Autodesk Inventor part; units mm, degrees
ref_plane "YZ Plane" through (0, 0, 0) normal (1, 0, 0) x (0, 1, 0)
ref_plane "XZ Plane" through (0, 0, 0) normal (0, 1, 0) x (-1, 0, 0)
ref_plane "XY Plane" through (0, 0, 0) normal (0, 0, 1) x (1, 0, 0)
sketch "Sketch1" plane through (0, 0, 0) normal (0, 0, 1) x (1, 0, 0)
  line L0 (35.093, -7.2202) -> (-19.907, -7.2202)
  line L1 (-19.907, -7.2202) -> (-19.907, 74.7798)
  line L2 (-19.907, 74.7798) -> (35.093, 74.7798)
  line L3 (35.093, 74.7798) -> (35.093, -7.2202)
  line L4 (-1.6316, 73.7798) -> (15.8684, 73.7798)
  line L5 (15.8684, 73.7798) -> (15.8684, 38.2798)
  line L6 (15.8684, 38.2798) -> (-1.6316, 38.2798)
  line L7 (-1.6316, 38.2798) -> (-1.6316, 73.7798)
  circle A0 centre (7.5885, 28.2798) radius 5.75
  line L8 (12.233, 6.0025) -> (3.233, 6.0025)
  line L9 (3.233, 6.0025) -> (3.233, -3.9975)
  line L10 (3.233, -3.9975) -> (12.233, -3.9975)
  line L11 (12.233, -3.9975) -> (12.233, 6.0025)
  circle A1 centre (7.5885, 28.2798) radius 1.25
  line L12 (3.233, 6.0025) -> (-2.767, 6.0025)
  line L13 (-2.767, 6.0025) -> (-2.767, -3.9975)
  line L14 (-2.767, -3.9975) -> (3.233, -3.9975)
  line L15 (3.233, -3.9975) -> (3.233, 6.0025)
  line L16 (12.233, 5.3167) -> (16.7288, 5.3167)
  line L17 (16.7288, 5.3167) -> (16.7288, 2.7767)
  line L18 (16.7288, 2.7767) -> (12.233, 2.7767)
  line L19 (12.233, 2.7767) -> (12.233, 5.3167)
  line L20 (12.233, -1.5375) -> (12.233, 1.0025)
  line L21 (12.233, -3.4895) -> (12.233, -0.9495)
  line L22 (12.233, 2.2687) -> (16.7288, 2.2687)
  line L23 (16.7288, 2.2687) -> (16.7288, -0.2713)
  line L24 (16.7288, -0.2713) -> (12.233, -0.2713)
  line L25 (12.233, -0.2713) -> (12.233, 2.2687)
  line L26 (12.233, -0.7793) -> (16.7288, -0.7793)
  line L27 (16.7288, -0.7793) -> (16.7288, -3.3193)
  line L28 (16.7288, -3.3193) -> (12.233, -3.3193)
  line L29 (12.233, -3.3193) -> (12.233, -0.7793)
  circle A2 centre (0.233, 0.9987) radius 1.5
  circle A3 centre (0.3684, 66.2798) radius 0.75
  circle A4 centre (0.3684, 63.7398) radius 0.75
  circle A5 centre (0.3684, 61.1998) radius 0.75
  circle A6 centre (0.3684, 58.6598) radius 0.75
  circle A7 centre (0.3684, 56.1198) radius 0.75
  circle A8 centre (0.3684, 53.5798) radius 0.75
  circle A9 centre (0.3684, 51.0398) radius 0.75
  circle A10 centre (0.3684, 48.4998) radius 0.75
  circle A11 centre (13.8684, 63.7398) radius 0.75
  circle A12 centre (13.8684, 58.6598) radius 0.75
  circle A13 centre (13.8684, 56.1198) radius 0.75
  circle A14 centre (13.8684, 53.5798) radius 0.75
  circle A15 centre (13.8684, 48.4998) radius 0.75
  circle A16 centre (13.8684, 66.2798) radius 0.75
  circle A17 centre (13.8684, 51.0398) radius 0.75
  circle A18 centre (13.8684, 61.1998) radius 0.75
  line L30 (-17.907, 69.7798) -> (-16.407, 69.7798)
  line L31 (-16.407, 69.7798) -> (-16.407, -2.2202)
  line L32 (-16.407, -2.2202) -> (-17.907, -2.2202)
  line L33 (-17.907, -2.2202) -> (-17.907, 69.7798)
  line L34 (-15.367, -2.2202) -> (-13.867, -2.2202)
  line L35 (-13.867, -2.2202) -> (-13.867, 69.7798)
  line L36 (-13.867, 69.7798) -> (-15.367, 69.7798)
  line L37 (-15.367, 69.7798) -> (-15.367, -2.2202)
  line L38 (31.593, 69.7798) -> (33.093, 69.7798)
  line L39 (33.093, 69.7798) -> (33.093, -2.2202)
  line L40 (33.093, -2.2202) -> (31.593, -2.2202)
  line L41 (31.593, -2.2202) -> (31.593, 69.7798)
  line L42 (30.553, -2.2202) -> (29.053, -2.2202)
  line L43 (29.053, -2.2202) -> (29.053, 69.7798)
  line L44 (29.053, 69.7798) -> (30.553, 69.7798)
  line L45 (30.553, 69.7798) -> (30.553, -2.2202)
  line L46 (5.8684, 68.7798) -> (10.8684, 68.7798)
  line L47 (10.8684, 68.7798) -> (10.8684, 63.7798)
  line L48 (10.8684, 63.7798) -> (5.8684, 63.7798)
  line L49 (5.8684, 63.7798) -> (5.8684, 68.7798)
  line L50 (6.8684, 55.8198) -> (10.8684, 55.8198)
  line L51 (10.8684, 55.8198) -> (10.8684, 53.2798)
  line L52 (10.8684, 53.2798) -> (6.8684, 53.2798)
  line L53 (6.8684, 53.2798) -> (6.8684, 55.8198)
  line L54 (5.8684, 48.2798) -> (10.8684, 48.2798)
  line L55 (10.8684, 48.2798) -> (10.8684, 43.2798)
  line L56 (10.8684, 43.2798) -> (5.8684, 43.2798)
  line L57 (5.8684, 43.2798) -> (5.8684, 48.2798)
  circle A19 centre (0.8684, 71.2798) radius 1.5
  circle A20 centre (0.8684, 40.7798) radius 1.5
  point P0 (0, 0)
  point P1 (0, 0)
  dimension "d0" = 82
  dimension "d1" = 55
  dimension "d2" = 17.5
  dimension "d3" = 35.5
  dimension "d4" = 11.5
  dimension "d5" = 2.5
  dimension "d6" = 1
  dimension "d7" = 10
  dimension "d8" = 27.4955
  dimension "d9" = 9
  dimension "d10" = 10
  dimension "d11" = 6
  dimension "d12" = 22.86
  dimension "d13" = 19.2246
  dimension "d14" = 2.54
  dimension "d15" = 0.6858
  dimension "d16" = 10
  dimension "d17" = 2.54
  dimension "d18" = 0.508
  dimension "d19" = 4.4958
  dimension "d20" = 4.4958
  dimension "d21" = 2.54
  dimension "d22" = 4.4958
  dimension "d23" = 0.508
  dimension "d24" = 3
  dimension "d25" = 1.5
  dimension "d26" = 7.5
  dimension "d27" = 2
  dimension "d28" = 1.5
  dimension "d29" = 1.5
  dimension "d30" = 1.5
  dimension "d31" = 1.5
  dimension "d32" = 1.5
  dimension "d33" = 1.5
  dimension "d34" = 1.5
  dimension "d35" = 2.54
  dimension "d36" = 2.54
  dimension "d37" = 2.54
  dimension "d38" = 2.54
  dimension "d39" = 2.54
  dimension "d40" = 2.54
  dimension "d41" = 2.54
  dimension "d42" = 1.5
  dimension "d43" = 1.5
  dimension "d44" = 1.5
  dimension "d45" = 1.5
  dimension "d46" = 1.5
  dimension "d47" = 1.5
  dimension "d48" = 1.5
  dimension "d49" = 1.5
  dimension "d50" = 2.54
  dimension "d51" = 2.54
  dimension "d52" = 2.54
  dimension "d53" = 2.54
  dimension "d54" = 2.54
  dimension "d55" = 2.54
  dimension "d56" = 2.54
  dimension "d57" = 2
  dimension "d58" = 7.5
  dimension "d59" = 2
  dimension "d60" = 2
  dimension "d61" = 2
  dimension "d62" = 2
  dimension "d63" = 2
extrude "Extrusion1" add sketch "Sketch1" along normal blind 2 contours L46 L47 L48 L49 | L50 L51 L52 L53 | L54 L55 L56 L57
fillet "Fillet1" radius 0.127 12 edges at (8.3684, 68.7798, 0) (5.8684, 66.2798, 0) (8.3684, 63.7798, 0) (10.8684, 66.2798, 0) (6.8684, 54.5498, 0) (8.8684, 55.8198, 0) (10.8684, 54.5498, 0) (8.8684, 53.2798, 0) (8.3684, 48.2798, 0) (5.8684, 45.7798, 0) (8.3684, 43.2798, 0) (10.8684, 45.7798, 0)
extrude "Extrusion2" add sketch "Sketch1" against normal blind 1.6 contours L4 L5 L6 L7 | L46 L47 L48 L49 | L50 L51 L52 L53 | L54 L55 L56 L57
properties part number "IMU"
CAD build for the part. Positions are in the model's coordinates, mm. A direction names the side the tool comes from. Coordinates: 2 decimals unless noted, no trailing zeros. Order: outer loops, then holes, each group sorted by start corner. A loop starts at its lowest first (then second) coordinate and runs counter-clockwise, first axis right, second up. Notation, with made-up numbers: (30.25, 10) - (60.25, 10) arc R23 cw to (60.25, 35) - close; hole circle Ø7 at (66, 7). An arc over 180 degrees is marked (long way). Answer in a Markdown table with one row per item.
1. 3-axis set-ups, long thin cutter, end or side, ignore diameter. For faces 1 (the face through (10.868, 55, 1)), 2 (the face through (8, 63.78, 1)), 3 (the face through (15.868, 56, -1)): which of +Z, -Z, +X, -X, +Y, -Y reach the whole face in a straight line?
Answer:
| item | result |
|---|---|
| face 1 | +Z, +X, +Y, -Y |
| face 2 | +Z, +X, -X |
| face 3 | +Z, -Z, +X, +Y, -Y |
2. Slice it at D-D, the plane z = -1. Give the number of separate pieces and of enclosed holes in the cut face, then the cut area to 3 significant figures.
Answer:
| item | result |
|---|---|
| separate pieces | 1 |
| enclosed holes | 18 |
| area | 579 mm² |
3. Drill centre lines: L1, parallel to Y at x = 9, z = 0.45; L2, parallel to Y at x = 6.5, z = 1.4; L3, parallel to Z at x = 13, y = 53.5. Where is each one in solid material? Low to high. Write a range as from..to.
Answer:
| item | result |
|---|---|
| L1 | 43.28..48.28, 53.28..55.82, 63.78..68.78 |
| L2 | 43.28..48.28, 63.78..68.78 |
| L3 | -1.6..0 |
4. Pull direction Y, two halves, no side cores. Call faces 4 (the face through (14, 63, -1)), 5 (the face through (5.868, 46, 1)), 6 (the face through (8, 68.78, 1)): +Y half, -Y half, draft (parallel to the pull), parting line (faces both ways), or undercut.
Answer:
| item | result |
|---|---|
| face 4 | undercut |
| face 5 | draft |
| face 6 | +Y half |
5. Slice it at A-A, the plane z = 0.45. List the corners of the cut face in (x, y).
Answer:
| item | result |
|---|---|
| outline | (5.87, 43.28) - (10.87, 43.28) - (10.87, 48.28) - (5.87, 48.28) - close; (5.87, 63.78) - (10.87, 63.78) - (10.87, 68.78) - (5.87, 68.78) - close; (6.87, 53.28) - (10.87, 53.28) - (10.87, 55.82) - (6.87, 55.82) - close |
6. Slice it at C-C, the plane y = 44. List the corners of the cut face in (x, z).
Answer:
| item | result |
|---|---|
| outline | (-1.63, -1.6) - (15.87, -1.6) - (15.87, 0) - (10.74, 0) arc R0.13 ccw to (10.87, 0.13) - (10.87, 2) - (5.87, 2) - (5.87, 0.13) arc R0.13 ccw to (6, 0) - (-1.63, 0) - close |
7. Slice it at B-B, the plane x = 10. List the corners of the cut face in (y, z), then the cut area to 3 significant figures.
Answer:
| item | result |
|---|---|
| outline | (38.28, -1.6) - (73.78, -1.6) - (73.78, 0) - (68.65, 0) arc R0.13 ccw to (68.78, 0.13) - (68.78, 2) - (63.78, 2) - (63.78, 0.13) arc R0.13 ccw to (63.91, 0) - (55.69, 0) arc R0.13 ccw to (55.82, 0.13) - (55.82, 2) - (53.28, 2) - (53.28, 0.13) arc R0.13 ccw to (53.41, 0) - (48.15, 0) arc R0.13 ccw to (48.28, 0.13) - (48.28, 2) - (43.28, 2) - (43.28, 0.13) arc R0.13 ccw to (43.41, 0) - (38.28, 0) - close |
| area | 81.9 mm² |
8. Flat gauge pins, fed straight in: P1, Ø2, axis at x = 0.37, y = 63.74, coming from the +Z side; P2, Ø0.9, axis at x = 13.87, y = 56.12, coming from the +Z side; P3, Ø2, axis at y = 43, z = 1.5, coming from the +X side; P4, Ø2, axis at x = 7.5, z = 1.5, coming from the -Y side. Where does each tip first touch, or does it go through?
Answer:
| item | result |
|---|---|
| P1 | z = 0 |
| P2 | through |
| P3 | x = 10.87 |
| P4 | y = 43.28 |
